from build123d import *


with BuildPart() as part:
    # Sketch1 → Revolve1 (revolve)
    with BuildSketch(Plane.XY):
        with BuildLine():
            Line((0, 0), (12.7, 0))
            ThreePointArc((12.7, 0), (18.686592918, 0.271905112), (24.623888889, 1.085381429))
            ThreePointArc((24.623888889, 1.085381429), (36.566761948, 8.064677779), (41.275, 21.071417912))
            Line((41.275, 21.071417912), (41.275, 68.602618404))
            ThreePointArc((41.275, 68.602618404), (40.018407707, 69.89932214), (38.734934185, 68.629219589))
            Line((38.734934185, 68.629219589), (38.734934185, 21.023040538))
            ThreePointArc((38.734934185, 21.023040538), (34.599795979, 9.671946754), (24.165277778, 3.583635989))
            ThreePointArc((24.165277778, 3.583635989), (18.456339345, 2.801447223), (12.7, 2.54))
            Line((12.7, 2.54), (0, 2.54))
            Line((0, 2.54), (0, 0))
        make_face()
    revolve(axis=Axis((0, 0, 0), (0, 1, 0)))


solid = part.part
Input: part model. Units: mm. Frame: model coordinates. Coordinates: 2 decimals unless noted, no trailing zeros. Write each loop counter-clockwise with the first axis right and the second up, starting at its lowest first coordinate (ties: lowest second). Pieces come first, ordered by that corner, then holes. Notation, with made-up numbers: M 40,-15.75 L 97,-15.75 A10 cw 97,-10.75 Z; hole C -31.5,11 d4. An arc over 180 degrees is marked long. Answer as a JSON object with one key per item and string values. Group by question number.
(1) Contact query for flat-ended pins moving along their axis: P1, Ø5, axis at x = 30.5, z = 19, coming from the -Y side; P2, Ø1.5, axis at x = -14, y = 15.5, coming from the +Z side; P3, Ø8, axis at y = 34.5, z = -7.5, coming from the +X side. Output: stop coordinate, or through.
(2) Section B-B on y = 16. Output: boundary loops of the cut face in (x, z), plus the area to 3 significant figures.
(3) Section A-A on y = 65.5. Output: boundary loops of the cut face in (x, z) (3 decimals), plus the area to 3 significant figures.
(4) Ray query, line 1 along Z through (x, y) = (0, 59) (3 decimals); line 2 along X through (y, z) = (29, -2). Return the intervals inside material, ascending. Write a range as [from, to].
(5) Mould query, pull axis X, two halves, no side actions, for faces 1 (the face through (0, 2.54, 0)), 2 (the face through (-8.948, 45.17, 40.293)), 3 (the face through (0, 0, 0)). Classes: pulls with the +X half, pulls with the -X half, needs draft (parallel to the pull), parting line crosses it, or undercut.
Result set:
{
 "1": {"P1": "stops at y = 5.03", "P2": "stops at z = 38.35", "P3": "stops at x = 41.13"},
 "2": {"outline": "C 0,0 d81.26; hole C 0,0 d75.99", "area": "651 mm2"},
 "3": {"outline": "C 0,0 d82.55; hole C 0,0 d77.47", "area": "638 mm2"},
 "4": {"line 1": "z = [-41.275, -38.735], [38.735, 41.275]", "line 2": "x = [-41.23, -38.68], [38.68, 41.23]"},
 "5": {"face 1": "undercut", "face 2": "parting line crosses it", "face 3": "needs draft"}
}
